```python
from build123d import *

# Parameters (mm, degrees)
F1_DEPTH = 12.7
F3_DEPTH = 25.4
F4_DEPTH = 25.4
F5_R     = 9.525927
F5_R_2   = 15.499369
F5_R_3   = 13.150127
F5_R_4   = 19.204473
F5_R_5   = 8.319425
F6_DEPTH = 25.4
F7_R     = 14.492161
F7_R_2   = 10.279788
F8_DEPTH = 25.4


with BuildPart() as f1:
    # F0 (on Front) → F1 (new body)
    with BuildSketch(Plane.XZ):
        with BuildLine():
            Line((-64.870612, 30.334717), (-55.738205, 25.88222))
            ThreePointArc((-55.738205, 25.88222), (-58.558762, 18.64157), (-60.443056, 11.102871))
            Line((-60.443056, 11.102871), (-70.559211, 10.16))
            Line((-70.559211, 10.16), (-70.559211, 0))
            Line((-70.559211, 0), (-70.559211, -10.16))
            Line((-70.559211, -10.16), (-60.443056, -11.102871))
            ThreePointArc((-60.443056, -11.102871), (-58.558762, -18.64157), (-55.738205, -25.88222))
            Line((-55.738205, -25.88222), (-64.870612, -30.334717))
            Line((-64.870612, -30.334717), (-55.965618, -48.599532))
            Line((-55.965618, -48.599532), (-44.09037, -42.809766))
            ThreePointArc((-44.09037, -42.809766), (-41.628099, -45.207722), (-39.035619, -47.464273))
            Line((-39.035619, -47.464273), (-44.09037, -56.27762))
            Line((-44.09037, -56.27762), (-26.463675, -66.387122))
            Line((-26.463675, -66.387122), (-21.423516, -57.599216))
            ThreePointArc((-21.423516, -57.599216), (-15.863285, -59.371651), (-10.16, -60.608672))
            Line((-10.16, -60.608672), (-10.16, -70.768672))
            Line((-10.16, -70.768672), (0, -70.768672))
            Line((0, -70.768672), (10.16, -70.768672))
            Line((10.16, -70.768672), (10.16, -60.608672))
            ThreePointArc((10.16, -60.608672), (15.863285, -59.371651), (21.423516, -57.599216))
            Line((21.423516, -57.599216), (26.463675, -66.387122))
            Line((26.463675, -66.387122), (44.09037, -56.27762))
            Line((44.09037, -56.27762), (39.035619, -47.464273))
            ThreePointArc((39.035619, -47.464273), (41.628099, -45.207722), (44.09037, -42.809766))
            Line((44.09037, -42.809766), (55.965618, -48.599532))
            Line((55.965618, -48.599532), (64.870612, -30.334717))
            Line((64.870612, -30.334717), (55.738205, -25.88222))
            ThreePointArc((55.738205, -25.88222), (58.558762, -18.64157), (60.443056, -11.102871))
            Line((60.443056, -11.102871), (70.559211, -10.16))
            Line((70.559211, -10.16), (70.559211, 0))
            Line((70.559211, 0), (70.559211, 10.16))
            Line((70.559211, 10.16), (60.443056, 11.102871))
            ThreePointArc((60.443056, 11.102871), (58.558762, 18.64157), (55.738205, 25.88222))
            Line((55.738205, 25.88222), (64.870612, 30.334717))
            Line((64.870612, 30.334717), (55.965618, 48.599532))
            Line((55.965618, 48.599532), (44.09037, 42.809766))
            ThreePointArc((44.09037, 42.809766), (41.628099, 45.207722), (39.035619, 47.464273))
            Line((39.035619, 47.464273), (44.09037, 56.27762))
            Line((44.09037, 56.27762), (26.463675, 66.387122))
            Line((26.463675, 66.387122), (21.423516, 57.599216))
            ThreePointArc((21.423516, 57.599216), (15.863285, 59.371651), (10.16, 60.608672))
            Line((10.16, 60.608672), (10.16, 70.768672))
            Line((10.16, 70.768672), (0, 70.768672))
            Line((0, 70.768672), (-10.16, 70.768672))
            Line((-10.16, 70.768672), (-10.16, 60.608672))
            ThreePointArc((-10.16, 60.608672), (-15.863285, 59.371651), (-21.423516, 57.599216))
            Line((-21.423516, 57.599216), (-26.463675, 66.387122))
            Line((-26.463675, 66.387122), (-44.09037, 56.27762))
            Line((-44.09037, 56.27762), (-39.035619, 47.464273))
            ThreePointArc((-39.035619, 47.464273), (-41.628099, 45.207722), (-44.09037, 42.809766))
            Line((-44.09037, 42.809766), (-55.965618, 48.599532))
            Line((-55.965618, 48.599532), (-64.870612, 30.334717))
        make_face()
    extrude(amount=F1_DEPTH)

    # F2 (on face) → F3 (cut)
    with BuildSketch(Plane.XZ.offset(12.7)):
        with BuildLine():
            ThreePointArc((-52.337367, 0), (-31.610057, -20.72731), (-10.882746, 0))
            ThreePointArc((-10.882746, 0), (-31.610057, 20.72731), (-52.337367, 0))
        make_face()
    extrude(amount=-F3_DEPTH, mode=Mode.SUBTRACT)

    # F2 (on face) → F4 (cut)
    with BuildSketch(Plane.XZ.offset(12.7)):
        with BuildLine():
            ThreePointArc((-52.337367, 0), (-31.610057, -20.72731), (-10.882746, 0))
            ThreePointArc((-10.882746, 0), (-31.610057, 20.72731), (-52.337367, 0))
        make_face()
    extrude(amount=-F4_DEPTH, mode=Mode.SUBTRACT)

    # F5 (on face) → F6 (cut)
    with BuildSketch(Plane.XZ.offset(12.7)):
        with Locations((-23.951983, 36.485761)):
            Circle(F5_R)
        with Locations((8.722895, 42.809766)):
            Circle(F5_R_2)
        with Locations((-23.76237, -36.997106)):
            Circle(F5_R_3)
        with Locations((12.633157, -37.899476)):
            Circle(F5_R_4)
        with Locations((7.218948, 3.308684)):
            Circle(F5_R_5)
    extrude(amount=-F6_DEPTH, mode=Mode.SUBTRACT)

    # F7 (on face) → F8 (cut)
    with BuildSketch(Plane.XZ.offset(12.7)):
        with Locations((39.102633, 18.348159)):
            Circle(F7_R)
        with Locations((34.590792, -9.926053)):
            Circle(F7_R_2)
    extrude(amount=-F8_DEPTH, mode=Mode.SUBTRACT)


solid = f1.part
```
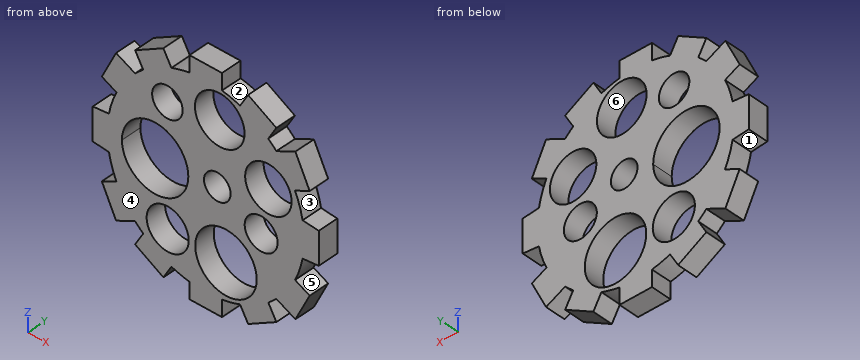
Can you work these out from the model? Positions are in its coordinate system, mm. Face numbers are marked on the shaded views. A direction names the side the tool comes from. Coordinates: 2 decimals unless noted, no trailing zeros. Loops run counter-clockwise (first coordinate to the right, second up) from the corner with the lowest first, then second, coordinate; pieces in that order, holes last. Notation, with made-up numbers: (6.25, 80) - (54.25, 80) arc R23 cw to (54.25, 106) - close; hole circle Ø3 at (60.25, 84). An arc over 180 degrees is marked (long way). Use a Markdown table: item, result.
Item 1: For the marked faces 1, 2 and 3, which set-ups out of +Z, -Z, +X, -X, +Y, -Y let a thin tool reach every point of the face, with its end or its side?
Numbers:
| item | result |
|---|---|
| face 1 | -X, +Y, -Y |
| face 2 | +Z, +Y, -Y |
| face 3 | +X, +Y, -Y |
Item 2: I want a section at D-D on y = -6. Give the number of separate pieces and of enclosed holes in the cut face, and give its area (3 significant figures).
Numbers:
| item | result |
|---|---|
| separate pieces | 1 |
| enclosed holes | 8 |
| area | 9,040 mm2 |
Item 3: I want a section at C-C on x = 41.5. Please give me the cut outline in (y, z), and give its area (3 significant figures).
Numbers:
| item | result |
|---|---|
| outline | (-12.7, -57.76) - (0, -57.76) - (0, -51.76) - (-12.7, -51.76) - close; (-12.7, -45.33) - (0, -45.33) - (0, -17.54) - (-12.7, -17.54) - close; (-12.7, -2.31) - (0, -2.31) - (0, 4.06) - (-12.7, 4.06) - close; (-12.7, 32.64) - (0, 32.64) - (0, 45.33) - (-12.7, 45.33) - close; (-12.7, 51.76) - (0, 51.76) - (0, 57.76) - (-12.7, 57.76) - close |
| area | 747 mm2 |
Item 4: Will these pins go through, and if not, where does the flat tip stop? pin 1 (5 mm diameter, centred on y = -7.5, z = 65.5, fed in from +X); pin 2 (3 mm diameter, centred on x = 52.5, y = -3, fed in from -Z); pin 3 (1.5 mm diameter, centred on x = -37, y = -3, fed in from +Z).
Numbers:
| item | result |
|---|---|
| pin 1 | stops at x = 32.37 |
| pin 2 | stops at z = -47.64 |
| pin 3 | stops at z = 60.77 |
Item 5: If I drill on probe 1 along Z at (x, y) = (16, -2); probe 2 along Z at (x, y) = (-23, -8); probe 3 along X at (y, z) = (-9.25, 64), over which ranges is the centre line in solid material (lowest first)? Write a range as from..to.
Numbers:
| item | result |
|---|---|
| probe 1 | z = -59.33..-56.81, -18.99..29.12, 56.49..59.33 |
| probe 2 | z = -60.35..-50.13, -23.87..-18.85, 18.85..27.01, 45.96..60.35 |
| probe 3 | x = -30.63..-25.09, -10.16..10.16, 25.09..30.63 |
Item 6: We'd pull the mould along X, two halves only. Please class the marked faces 4, 5 and 6: released by +X, released by -X, zero draft, split by the parting line, or undercut.
Numbers:
| item | result |
|---|---|
| face 4 | zero draft |
| face 5 | released by +X |
| face 6 | undercut |
Item 7: I want a section at A-A on x = 3.5. Please give me the cut outline in (y, z), and give its area (3 significant figures).
Numbers:
| item | result |
|---|---|
| outline | (-12.7, -70.77) - (0, -70.77) - (0, -54.79) - (-12.7, -54.79) - close; (-12.7, -21.01) - (0, -21.01) - (0, -4.13) - (-12.7, -4.13) - close; (-12.7, 10.75) - (0, 10.75) - (0, 28.22) - (-12.7, 28.22) - close; (-12.7, 57.4) - (0, 57.4) - (0, 70.77) - (-12.7, 70.77) - close |
| area | 809 mm2 |
Item 8: I want a section at B-B on z = -52. Please give me the cut outline in (x, y).
Numbers:
| item | result |
|---|---|
| outline | (-41.64, -12.7) - (-0.4, -12.7) - (-0.4, 0) - (-41.64, 0) - close; (25.67, -12.7) - (41.64, -12.7) - (41.64, 0) - (25.67, 0) - close |
